from build123d import *

# Parameters (mm, degrees)
F0_W     = 10
F0_H     = 7.5
F1_DEPTH = 20
F2_R     = 5
F3_R     = 9.99999
F4_R     = 5


# Not quite as in the source:
# - a fillet or chamfer is up to 0.001 mm smaller than in the source, because OpenCascade refuses the exact size


with BuildPart() as f1:
    # F0 (on Front) → F1 (new body)
    with BuildSketch(Plane.XZ):
        with Locations((5, 3.75)):
            Rectangle(F0_W, F0_H)
        Polygon((10, 7.5), (10, 0), (22.0492679997, 14.3597584268), (21.6662457782, 14.6811522316), (22.3090333878, 15.4471966748), (22.6920556094, 15.1258028699), (23.3348432191, 15.891847313), (22.9518209975, 16.2132411179), (23.5946086072, 16.979285561), (23.9776308288, 16.6578917562), (24.6204184385, 17.4239361993), (24.2373962169, 17.7453300041), (24.8801838266, 18.5113744472), (25.2632060482, 18.1899806424), (25.9059936578, 18.9560250855), (25.5229714363, 19.2774188904), (26.165759046, 20.0434633335), (26.5487812675, 19.7220695286), (27.1915688772, 20.4881139717), (26.8085466557, 20.8095077766), (27.4513342653, 21.5755522197), (27.8343564869, 21.2541584149), (32.9766573644, 27.3825139598), (29.2836282906, 30.4813332936), (24.1413274131, 24.3529777486), (24.5243496347, 24.0315839438), (23.881562025, 23.2655395007), (23.4985398034, 23.5869333055), (22.8557521937, 22.8208888624), (23.2387744153, 22.4994950575), (22.5959868056, 21.7334506144), (22.212964584, 22.0548444193), (21.5701769744, 21.2887999761), (21.9531991959, 20.9674061713), (21.3104115862, 20.2013617282), (20.9273893647, 20.522755533), (20.284601755, 19.7567110899), (20.6676239765, 19.4353172851), (20.0248363669, 18.6692728419), (19.6418141453, 18.9906666468), (18.9990265356, 18.2246222037), (19.3820487572, 17.9032283988), (18.7392611475, 17.1371839557), (18.3562389259, 17.4585777605), align=None)
    extrude(amount=F1_DEPTH)

    # F2
    f2_edges = [f1.edges().sort_by_distance(p)[0] for p in [
        (10, -10, 7.5),
    ]]
    fillet(f2_edges, radius=F2_R)

    # F3 (radius 10 in the source; OpenCascade refuses exactly that, so slightly less here)
    f3_edges = [f1.edges().sort_by_distance(p)[0] for p in [
        (31.130143, -20, 28.931924),
        (31.130143, 0, 28.931924),
    ]]
    fillet(f3_edges, radius=F3_R)

    # F4
    f4_edges = [f1.edges().sort_by_distance(p)[0] for p in [
        (10, -10, 0),
    ]]
    fillet(f4_edges, radius=F4_R)


solid = f1.part
CAD build for the part. Positions are in the model's coordinates, mm. A direction names the side the tool comes from. Coordinates: 2 decimals unless noted, no trailing zeros. Write each loop counter-clockwise with the first axis right and the second up, starting at its lowest first coordinate (ties: lowest second). Pieces come first, ordered by that corner, then holes. Notation, with made-up numbers: M 66,27.5 L 101,27.5 A20 cw 101,61.5 Z; hole C 30,52.25 d9. An arc over 180 degrees is marked long. Answer as a JSON object with one key per item and string values. Group by question number.
1) Tool access for faces 1 (the face through (4, -10, 7.5)), 2 (the face through (29.17, -17.15, 26.65)): list every direction of +Z, -Z, +X, -X, +Y, -Y with a clear straight run to the whole face (end or side of a thin tool).
2) Saw through at A-A (z = 3). Write the cut outline in (x, y), plus the area to 3 significant figures.
3) Saw through at B-B (x = 17.5). Write the cut outline in (y, z).
4) Pin check, flat tips, straight feed: pin 1 Ø10 at (y, z) = (-12, 10.5) entering from +X; pin 2 Ø1.5 at (y, z) = (-16, 4.5) entering from +X; pin 3 Ø4 at (x, y) = (3.5, -11.5) entering from +Z; pin 4 Ø8 at (x, z) = (22.5, 3.5) entering from -Y. Stop position of each tip, or through.
5) Wall check: line 1 (Z direction, x = 5, y = -13.25); line 2 (Z direction, x = 18, y = -8.25); line 3 (X direction, y = -9.75, z = 25.5). Give the ranges that are in metal, low to high. Write a range as from..to.
Values follow:
{
 "1": {"face 1": "+Z, -X, +Y, -Y", "face 2": "+Z, +X, -Y"},
 "2": {"outline": "M 0,-20 L 12.52,-20 L 12.52,0 L 0,0 Z", "area": "250 mm2"},
 "3": {"outline": "M -20,8.94 L 0,8.94 L 0,16.44 L -20,16.44 Z"},
 "4": {"pin 1": "stops at x = 23.01", "pin 2": "stops at x = 14.41", "pin 3": "stops at z = 7.5", "pin 4": "passes through"},
 "5": {"line 1": "z = 0..7.5", "line 2": "z = 9.53..17.03", "line 3": "x = 25.1..31.4"}
}
